Geometry: see drawing. Coordinates: mm, zero at the bounding-box minimum. A direction names the side the tool comes from. Coordinates: 2 decimals unless noted, no trailing zeros. Write each loop counter-clockwise with the first axis right and the second up, starting at its lowest first coordinate (ties: lowest second). Pieces come first, ordered by that corner, then holes.
1) Section query A-A (y = 16). Output: boundary loops of the cut face in (x, z).
2) Set-up query: the marked faces 4 and 5. Return all of +Z, -Z, +X, -X, +Y, -Y with unobstructed straight access to the full face (end or side cutting, diameter ignored); none if empty.
3) Pin query (flat end, axial travel): pin 1 Ø2.5 at (x, y) = (24.49, 7.51) entering from -Z; pin 2 Ø2 at (x, z) = (24, 7) entering from +Y; pin 3 Ø3 at (y, z) = (22, 5.5) entering from -X (1 decimal); pin 4 Ø1 at (y, z) = (14, 9) entering from +X. Return the tip coordinate at first contact, or that it passes through.
4) Section query D-D (z = 12.5). Output: boundary loops of the cut face in (x, y).
5) Section query C-C (y = 23). Output: boundary loops of the cut face in (x, z).
6) Draft query along X for the marked faces 1, 2 and 3. Return one class per face: pulls with the +X half, pulls with the -X half, needs draft (parallel to the pull), parting line crosses it, or undercut.
7) Line query: L1, parallel to Y at x = 16, z = 11.5; L2, parallel to Z at x = 27.5, y = 9; L3, parallel to Y at x = 13, z = 14 (1 decimal). Output: solid intervals per line, ascending.
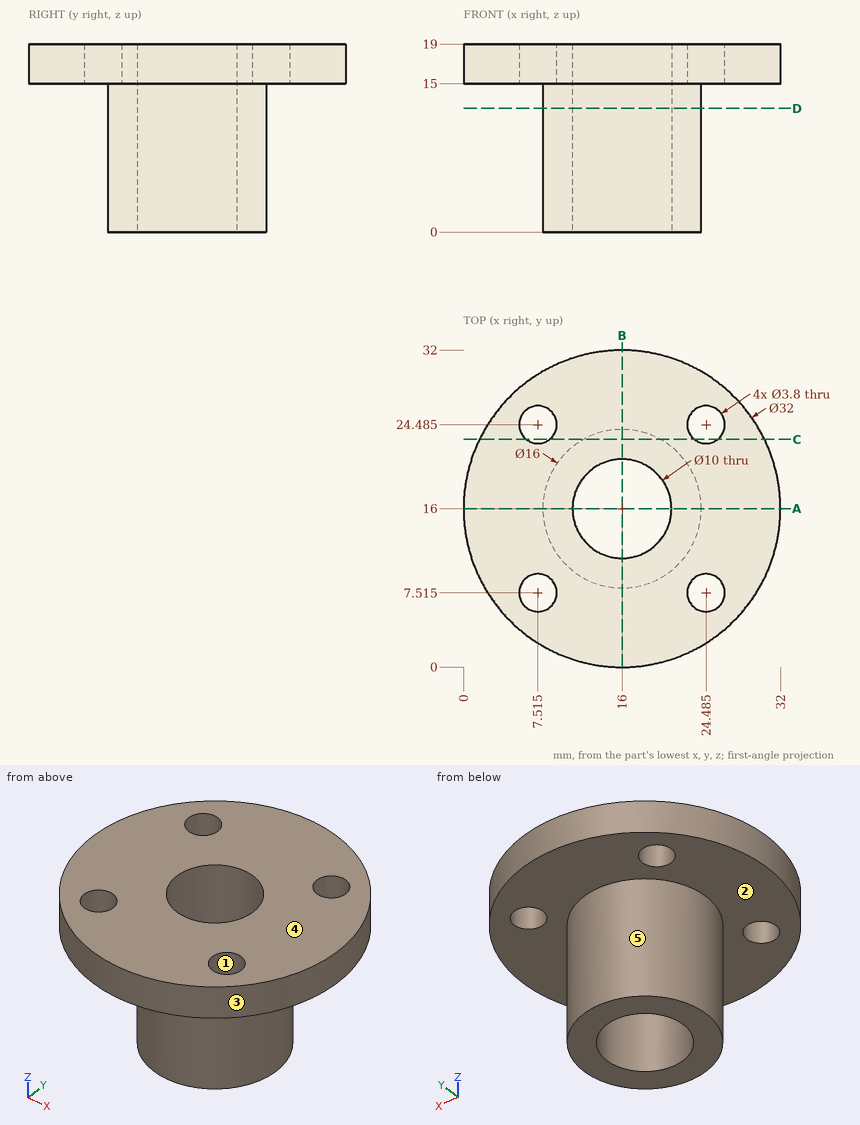
Answer:
1. outline: (0, 15) - (8, 15) - (8, 0) - (11, 0) - (11, 19) - (0, 19) - close; (21, 0) - (24, 0) - (24, 15) - (32, 15) - (32, 19) - (21, 19) - close
2. face 4: +Z, +X, -X, +Y, -Y
2. face 5: -Z
3. pin 1: passes through
3. pin 2: stops at y = 19.87
3. pin 3: stops at x = 9.4
3. pin 4: stops at x = 23.86
4. outline: circle Ø16 at (16, 16); hole circle Ø10 at (16, 16)
5. outline: (1.61, 15) - (6.33, 15) - (6.33, 19) - (1.61, 19) - close; (8.7, 15) - (12.13, 15) - (12.13, 0) - (19.87, 0) - (19.87, 15) - (23.3, 15) - (23.3, 19) - (8.7, 19) - close; (25.67, 15) - (30.39, 15) - (30.39, 19) - (25.67, 19) - close
6. face 1: undercut
6. face 2: needs draft
6. face 3: parting line crosses it
7. L1: y = 8 to 11, 21 to 24
7. L2: z = 15 to 19
7. L3: y = 8.6 to 12, 20 to 23.4
